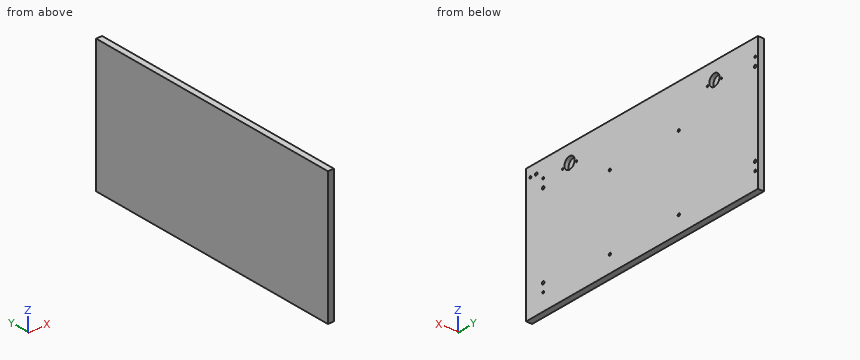
```python
from build123d import *

# Parameters (mm, degrees)
SKETCH1_W                      = 18
SKETCH1_H                      = 396
LEFT_HAND_END_DEPTH            = 800
SKETCH3_R                      = 3.75
SHELF_MOUNT_HOLES_DEPTH        = 8
SKETCH2_R                      = 3.25
SKETCH2_R_2                    = 4.25
BASE_AND_TOP_MOUNT_HOLES_DEPTH = 12
SKETCH4_R                      = 17.5
SKETCH4_R_2                    = 2.5
HINGE_HOLES_DEPTH              = 12


with BuildPart() as part:
    # Sketch1 → Left Hand End (new body)
    with BuildSketch(Plane(origin=(0, -800, 0), x_dir=(-1, 0, 0), z_dir=(0, 1, 0))):
        with Locations((9, -198)):
            Rectangle(SKETCH1_W, SKETCH1_H)
    extrude(amount=LEFT_HAND_END_DEPTH)

    # Sketch3 → Shelf Mount Holes (cut)
    with BuildSketch(Plane(origin=(0, 0, 0), x_dir=(0, 0, -1), z_dir=(1, 0, 0))):
        with Locations((128, -511)):
            Circle(SKETCH3_R)
        with Locations((346, -511)):
            Circle(SKETCH3_R)
        with Locations((346, -273)):
            Circle(SKETCH3_R)
        with Locations((128, -273)):
            Circle(SKETCH3_R)
    extrude(amount=-SHELF_MOUNT_HOLES_DEPTH, mode=Mode.SUBTRACT)

    # Sketch2 → Base and Top Mount Holes (cut)
    with BuildSketch(Plane(origin=(0, 0, 0), x_dir=(0, 0, -1), z_dir=(1, 0, 0))):
        with Locations((50, -9)):
            Circle(SKETCH2_R)
        with Locations((346, -9)):
            Circle(SKETCH2_R)
        with Locations((75, -9)):
            Circle(SKETCH2_R_2)
        with Locations((321, -9)):
            Circle(SKETCH2_R_2)
        with Locations((50, -741)):
            Circle(SKETCH2_R)
        with Locations((75, -741)):
            Circle(SKETCH2_R_2)
        with Locations((321, -741)):
            Circle(SKETCH2_R_2)
        with Locations((346, -741)):
            Circle(SKETCH2_R)
        with Locations((29, -765)):
            Circle(SKETCH2_R_2)
        with Locations((29, -785)):
            Circle(SKETCH2_R)
    extrude(amount=-BASE_AND_TOP_MOUNT_HOLES_DEPTH, mode=Mode.SUBTRACT)

    # Sketch4 → Hinge Holes (cut)
    with BuildSketch(Plane(origin=(0, 0, 0), x_dir=(0, 0, -1), z_dir=(1, 0, 0))):
        with Locations((49.5, -650)):
            Circle(SKETCH4_R)
        with Locations((55.5, -626)):
            Circle(SKETCH4_R_2)
        with Locations((55.5, -674)):
            Circle(SKETCH4_R_2)
        with Locations((49.5, -150)):
            Circle(SKETCH4_R)
        with Locations((55.5, -126)):
            Circle(SKETCH4_R_2)
        with Locations((55.5, -174)):
            Circle(SKETCH4_R_2)
    extrude(amount=-HINGE_HOLES_DEPTH, mode=Mode.SUBTRACT)


solid = part.part
```
For this review, take the finished solid that the model builds, in its own axes (mm). Round coordinates to 2 decimals unless told otherwise and drop trailing zeros. Write each loop counter-clockwise with the first axis right and the second up, starting at its lowest first coordinate (ties: lowest second). Pieces come first, ordered by that corner, then holes. Notation, with made-up numbers: (89, 87) -> (115, 87) arc R30 cw to (115, 122) -> close; hole circle Ø1 at (32.5, 39). An arc over 180 degrees is marked (long way). One line per question, with ' | ' between items. Start each with the question number.
1) Wall thickness on line 1 along Y through (x, z) = (-9.5, -29); line 2 along Z through (x, y) = (-4.5, -273); line 3 along Y through (x, z) = (-9.25, -320.5): over which ranges is each line inside the solid? List them lowest first.
2) For pin 1 Ø21 at (y, z) = (-650, -49.5) entering from +X; pin 2 Ø7 at (y, z) = (-742.5, -320.5) entering from +X, all flat-tipped, find the tip position at first contact; note any pin that passes through.
3) Add section A-A (y = -150). Write out the cut boundary in (x, z).
Reported:
1) line 1: y = -800 to -788.25, -781.75 to -769.25, -760.75 to 0 | line 2: z = -396 to -349.75, -342.25 to -131.75, -124.25 to 0 | line 3: y = -800 to -745.22, -736.78 to -13.22, -4.78 to 0
2) pin 1: stops at x = -12 | pin 2: stops at x = 0
3) outline: (-18, -396) -> (0, -396) -> (0, -67) -> (-12, -67) -> (-12, -32) -> (0, -32) -> (0, 0) -> (-18, 0) -> close
